Source: CAD feature listing. Evaluate the final solid. Frame: model axes, mm. Give positions to 0.01 mm unless a question says otherwise; leave off trailing zeros. Write each loop counter-clockwise with the first axis right and the second up, starting at its lowest first coordinate (ties: lowest second). Pieces come first, ordered by that corner, then holes.
Autodesk Inventor part; units mm, degrees
ref_plane "YZ Plane" through (0, 0, 0) normal (1, 0, 0) x (0, 1, 0)
ref_plane "XZ Plane" through (0, 0, 0) normal (0, 1, 0) x (-1, 0, 0)
ref_plane "XY Plane" through (0, 0, 0) normal (0, 0, 1) x (1, 0, 0)
sketch "Sketch1" plane through (0, 0, 0) normal (0, 0, 1) x (1, 0, 0)
  circle A0 centre (0, 0) radius 141.5
  circle A1 centre (0, 0) radius 161.671
  dimension "d0" = 283
  dimension "d1" = 323.342
extrude "Extrusion1" add sketch "Sketch1" along normal blind 263
sketch "Sketch2" plane through (0, 0, 263) normal (0, 0, 1) x (1, 0, 0)
  circle A0 centre (0, 0) radius 161.671
  circle A1 centre (0, 0) radius 160.0835
  dimension "d4" = 320.167
extrude "Extrusion2" cut sketch "Sketch2" against normal blind 25.4
fillet "Fillet1" radius 0.7937 1 edges at (-160.0835, 0, 237.6)
chamfer "Chamfer1" distance 0.7937 angle 45 1 edges at (-161.671, 0, 0)
properties part number "A1-19027-400-09 HCWI liner - drain" material "Iron, HCWI"
1. Mould query, pull axis X, two halves, no side actions, for faces 1 (the cylindrical face through (-30.674, 138.135, 129.659)), 2 (the flat face through (-1, -142, 263)), 3 (the cylindrical face through (-159.93, 7.04, 250.87)). Classes: +X half, -X half, draft (parallel to the pull), parting line (faces both ways), or undercut.
2. Cut plane C-C, the plane z = 174. Return the cut outline in (x, y), then the cut area to 3 significant figures.
3. Contact query for flat-ended pins moving along their axis: P1, Ø3, axis at y = -56.5, z = 182.5, coming from the -X side; P2, Ø6, axis at x = 64.5, y = -120, coming from the +Z side; P3, Ø3, axis at x = 95, z = 144, coming from the -Y side; P4, Ø2, axis at y = -63.5, z = 63.5, coming from the +X side. Output: stop coordinate, or through.
4. Cut plane A-A, the plane y = 0. Return the cut outline in (x, z).
5. Line query: L1, parallel to Y at x = 0, z = 62; L2, parallel to X at y = -4, z = 88; L3, parallel to X at y = -2.5, z = 15.5. Output: solid intervals per line, ascending.
Response values:
1. face 1: undercut
1. face 2: draft
1. face 3: parting line
2. outline: circle Ø323.34 at (0, 0); hole circle Ø283 at (0, 0)
2. area: 19,200 mm2
3. P1: stops at x = -152.03
3. P2: passes through
3. P3: stops at y = -131.89
3. P4: stops at x = 149.1
4. outline: (-161.67, 0.79) - (-160.88, 0) - (-141.5, 0) - (-141.5, 263) - (-160.08, 263) - (-160.08, 238.39) arc R0.79 cw to (-160.88, 237.6) - (-161.67, 237.6) - close; (141.5, 0) - (160.88, 0) - (161.67, 0.79) - (161.67, 237.6) - (160.88, 237.6) arc R0.79 cw to (160.08, 238.39) - (160.08, 263) - (141.5, 263) - close
5. L1: y = -161.67 to -141.5, 141.5 to 161.67
5. L2: x = -161.62 to -141.44, 141.44 to 161.62
5. L3: x = -161.65 to -141.48, 141.48 to 161.65
